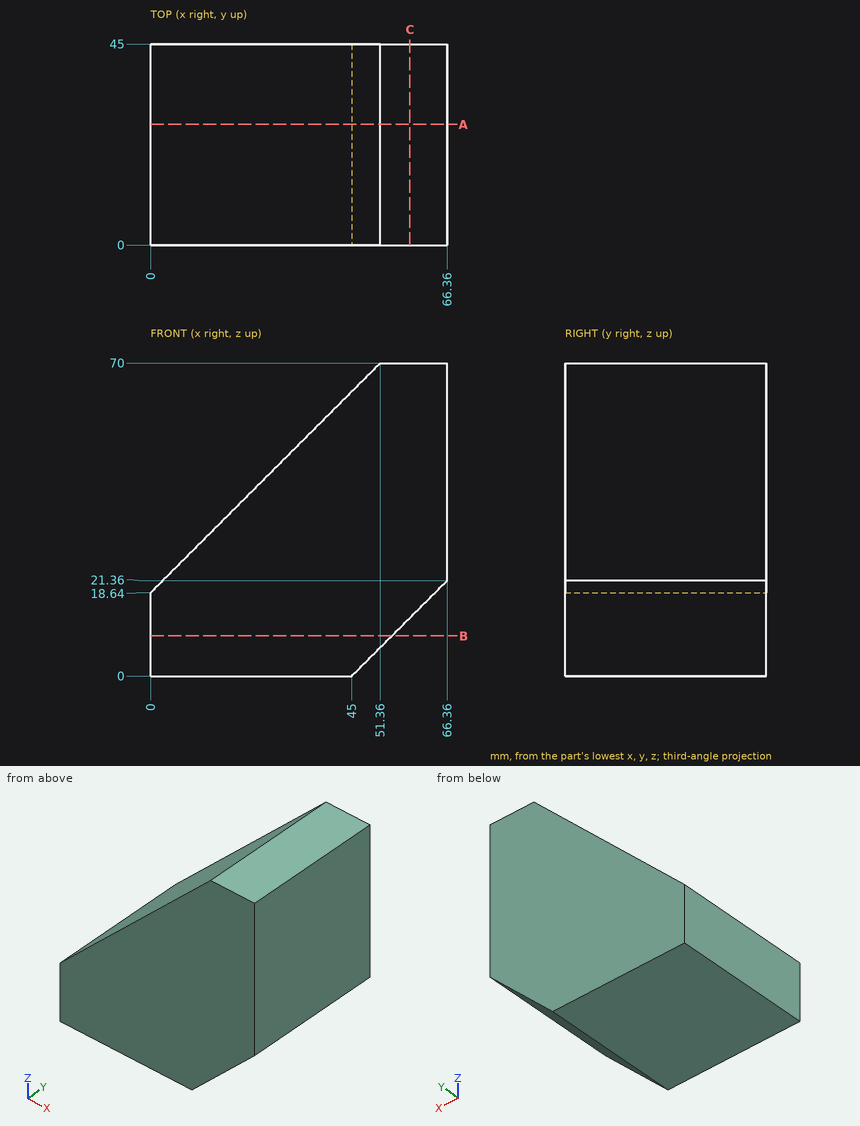
Design review of the part shown in the three views and the two pictorial views. Dimensions are in mm from the part's minimum x, y and z. Give positions to 0.01 mm unless a question says otherwise; leave off trailing zeros. Order: outer loops, then holes, each group sorted by start corner. A loop starts at its lowest first (then second) coordinate and runs counter-clockwise, first axis right, second up. Notation, with made-up numbers: (24.25, 73.25) -> (66.25, 73.25) arc R29 cw to (66.25, 96.25) -> close; hole circle Ø1 at (-34, 17). An arc over 180 degrees is marked (long way). Write each question's results on one line, items separated by ' | '. Start each with the question number.
Q1. Add section C-C on x = 58. Give the boundary of the cut face in (y, z), and give its area (4 significant figures).
Q2. Wall thickness on L1, parallel to X at y = 19, z = 19; L2, parallel to X at y = 5, z = 7; L3, parallel to Z at x = 59.5, y = 34: over which ranges is each line inside the solid? List them lowest first. Write a range as from..to.
Q3. Add section A-A on y = 27. Give the boundary of the cut face in (x, z), and give its area (3 significant figures).
Q4. Add section B-B on z = 9. Give the boundary of the cut face in (x, y).
Q5. For pin 1 (8 mm diameter, centred on x = 27.5, y = 38, fed in from +Z); pin 2 (8 mm diameter, centred on y = 29, z = 58, fed in from -X); pin 3 (1.5 mm diameter, centred on x = 15, y = 35, fed in from +Z), all flat-tipped, find the tip position at first contact; note any pin that passes through.
Found:
1) outline: (0, 13) -> (45, 13) -> (45, 70) -> (0, 70) -> close | area: 2,565 mm2
2) L1: x = 0.36..64 | L2: x = 0..52 | L3: z = 14.5..70
3) outline: (0, 0) -> (45, 0) -> (66.36, 21.36) -> (66.36, 70) -> (51.36, 70) -> (0, 18.64) -> close | area: 3,100 mm2
4) outline: (0, 0) -> (54, 0) -> (54, 45) -> (0, 45) -> close
5) pin 1: stops at z = 50.14 | pin 2: stops at x = 35.36 | pin 3: stops at z = 34.39
